Can you work these out from the model? Positions are in its coordinate system, mm. A direction names the side the tool comes from. Give positions to 0.01 mm unless a question says otherwise; leave off trailing zeros. Write each loop counter-clockwise with the first axis right and the second up, starting at its lowest first coordinate (ties: lowest second). Pieces come first, ordered by that corner, then holes.
1. Thinking about a two-plate mould opening in Z: for faces 3 (the cylindrical face through (5.949, -5.761, 45.005)), 4 (the flat face through (-2.3, -6.2, 60.325)), 5 (the flat face through (3.219, 5.474, 29.74)), 6 (the flat face through (-2.3, -6.2, 0)), which applies, pulls with the +Z half, pulls with the -Z half, needs draft (parallel to the pull), parting line crosses it, or undercut?
2. Suppose I cut it at A-A (y = 0). Please give me the cut outline in (x, z) (3 decimals), and give its area (3 significant figures).
3. Suppose I cut it at C-C (x = -4). Give the number of separate pieces and of enclosed holes in the cut face, and give its area (3 significant figures).
4. On a 3-axis mill with a long thin cutter (end or side, diameter ignored), from which of +Z, -Z, +X, -X, +Y, -Y can I reach the whole of each face in a straight line? I mean faces 1 (the flat face through (3.131, -5.525, 29.74)), 2 (the cylindrical face through (-6.02, 5.67, 45.62)). Say none if no direction works.
5. Suppose I cut it at B-B (z = 11). Please give me the cut outline in (x, y) (3 decimals), and give its area (3 significant figures).
6. If I drill on probe 1 along X at (y, z) = (-2.5, 8.5); probe 2 along X at (y, z) = (-0.5, 4.5); probe 3 along Z at (x, y) = (-4.25, 5) (3 decimals), over which ranges is the centre line in solid material (lowest first)?
7. I'm going to push flat-ended pins straight in: pin 1 (6 mm diameter, centred on x = -7.5, z = 9, fed in from +Y) (3 decimals); pin 2 (3 mm diameter, centred on y = -2, z = 32, fed in from -X); pin 3 (5 mm diameter, centred on x = 2, y = 6, fed in from -Z); pin 4 (2 mm diameter, centred on x = -7.5, z = 13.5, fed in from -Y). Where does each tip first touch, or does it pass through?
```python
from build123d import *

# Parameters (mm, degrees)
SKETCH1_R               = 9.525
BOSS_EXTRUDE1_DEPTH     = 60.325
SKETCH3_R               = 2.38125
CUT_EXTRUDE1_DEPTH      = 24.171391971
CUT_EXTRUDE1_DEPTH_BACK = 3.851391971


with BuildPart() as part:
    # Sketch1 → Boss-Extrude1 (new body)
    with BuildSketch(Plane.XY):
        Circle(SKETCH1_R)
        Polygon((6.35, 3.666174209), (0, 7.332348419), (-6.35, 3.666174209), (-6.35, -3.666174209), (0, -7.332348419), (6.35, -3.666174209), align=None, mode=Mode.SUBTRACT)
    extrude(amount=BOSS_EXTRUDE1_DEPTH)

    # Sketch3 → Cut-Extrude1 (cut, two sides)
    with BuildSketch(Plane(origin=(5.08, -8.798818102, 0), x_dir=(0.866025404, 0.5, 0), z_dir=(-0.5, 0.866025404, 0))) as cut_extrude1_sk:
        with Locations((0, -5.08)):
            Circle(SKETCH3_R)
        with Locations((0, -45.72)):
            Circle(SKETCH3_R)
    extrude(amount=CUT_EXTRUDE1_DEPTH, mode=Mode.SUBTRACT)
    extrude(cut_extrude1_sk.sketch, amount=-CUT_EXTRUDE1_DEPTH_BACK, mode=Mode.SUBTRACT)


solid = part.part
```
Checks:
1. face 3: undercut
1. face 4: pulls with the +Z half
1. face 5: needs draft
1. face 6: pulls with the -Z half
2. outline: (-9.525, 0) - (-6.35, 0) - (-6.35, 60.325) - (-9.525, 60.325) - close; (6.35, 0) - (9.525, 0) - (9.525, 60.325) - (6.35, 60.325) - close
2. area: 383 mm2
3. separate pieces: 4
3. enclosed holes: 0
3. area: 403 mm2
4. face 1: +Z, -Z
4. face 2: none
5. outline: circle Ø19.05 at (0, 0); hole (-6.35, -3.666) - (0, -7.332) - (6.35, -3.666) - (6.35, 3.666) - (0, 7.332) - (-6.35, 3.666) - close
5. area: 145 mm2
6. probe 1: x = -9.19 to -6.35, 6.35 to 9.19
6. probe 2: x = -9.51 to -6.35, 6.35 to 9.51
6. probe 3: z = 0 to 3.012, 7.148 to 43.652, 47.788 to 60.325
7. pin 1: stops at y = 8.395
7. pin 2: stops at x = -9.51
7. pin 3: stops at z = 0
7. pin 4: stops at y = -6.96
